Design review of the part built by this model. Coordinates are the model's own, in mm. Give positions to 0.01 mm unless a question says otherwise; leave off trailing zeros. Loops run counter-clockwise (first coordinate to the right, second up) from the corner with the lowest first, then second, coordinate; pieces in that order, holes last. Notation, with made-up numbers: (53.25, 64) - (100.25, 64) arc R19 cw to (100.25, 77) - close; hole circle Ø8 at (73.25, 37). An arc over 180 degrees is marked (long way). Write each question's results on one line, items separated by ' | '.
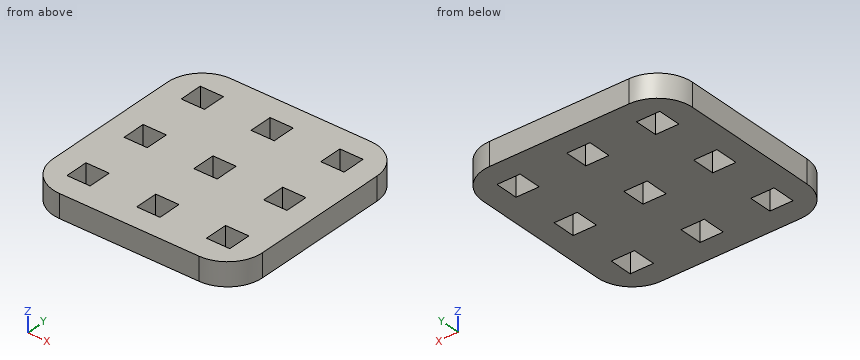
from build123d import *

# Parameters (mm, degrees)
MODEL_W                 = 3
MODEL_H                 = 3
SALIENTE_EXTRUIR1_DEPTH = 3


with BuildPart() as part:
    # Model → Saliente-Extruir1 (new body)
    with BuildSketch(Plane.XY):
        with BuildLine():
            Line((12.895467255, 298.259658236), (30.895467255, 298.259658236))
            ThreePointArc((30.895467255, 298.259658236), (34.077447771, 296.941638751), (35.395467255, 293.759658236))
            Line((35.395467255, 293.759658236), (35.395467255, 275.759658236))
            ThreePointArc((35.395467255, 275.759658236), (34.077447771, 272.577677721), (30.895467255, 271.259658236))
            Line((30.895467255, 271.259658236), (12.895467255, 271.259658236))
            ThreePointArc((12.895467255, 271.259658236), (9.71348674, 272.577677721), (8.395467255, 275.759658236))
            Line((8.395467255, 275.759658236), (8.395467255, 293.759658236))
            ThreePointArc((8.395467255, 293.759658236), (9.71348674, 296.941638751), (12.895467255, 298.259658236))
        make_face()
        with Locations((12.895467255, 293.759658236)):
            Rectangle(MODEL_W, MODEL_H, mode=Mode.SUBTRACT)
        with Locations((21.895467255, 293.759658236)):
            Rectangle(MODEL_W, MODEL_H, mode=Mode.SUBTRACT)
        with Locations((30.895467255, 293.759658236)):
            Rectangle(MODEL_W, MODEL_H, mode=Mode.SUBTRACT)
        with Locations((12.895467255, 275.759658236)):
            Rectangle(MODEL_W, MODEL_H, mode=Mode.SUBTRACT)
        with Locations((21.895467255, 275.759658236)):
            Rectangle(MODEL_W, MODEL_H, mode=Mode.SUBTRACT)
        with Locations((30.895467255, 275.759658236)):
            Rectangle(MODEL_W, MODEL_H, mode=Mode.SUBTRACT)
        with Locations((12.895467255, 284.759658236)):
            Rectangle(MODEL_W, MODEL_H, mode=Mode.SUBTRACT)
        with Locations((21.895467255, 284.759658236)):
            Rectangle(MODEL_W, MODEL_H, mode=Mode.SUBTRACT)
        with Locations((30.895467255, 284.759658236)):
            Rectangle(MODEL_W, MODEL_H, mode=Mode.SUBTRACT)
    extrude(amount=SALIENTE_EXTRUIR1_DEPTH)


solid = part.part
(1) Take a section at B-B on x = 20.75. Give the boundary of the cut face in (y, z), plus the area to 3 significant figures.
Answers below:
outline: (271.26, 0) - (274.26, 0) - (274.26, 3) - (271.26, 3) - close; (277.26, 0) - (283.26, 0) - (283.26, 3) - (277.26, 3) - close; (286.26, 0) - (292.26, 0) - (292.26, 3) - (286.26, 3) - close; (295.26, 0) - (298.26, 0) - (298.26, 3) - (295.26, 3) - close | area: 54.0 mm2
(2) Wall thickness on line 1 along Y through (x, z) = (22, 2.6); line 2 along X through (y, z) = (276.75, 2.25); line 3 along X through (y, z) = (274.5, 0.4): over which ranges is each line inside the solid? List them lowest first. Write a range as from..to.
Answers below:
line 1: 271.26..274.26, 277.26..283.26, 286.26..292.26, 295.26..298.26 | line 2: 8.4..11.4, 14.4..20.4, 23.4..29.4, 32.4..35.4 | line 3: 8.58..11.4, 14.4..20.4, 23.4..29.4, 32.4..35.22
(3) Take a section at C-C on z = 2.4. Count the separate pieces of the cut face and the enclosed holes in it, plus the area to 3 significant figures.
Answers below:
separate pieces: 1 | enclosed holes: 9 | area: 631 mm2
(4) Take a section at A-A on y = 285.5. Give the boundary of the cut face in (x, z).
Answers below:
outline: (8.4, 0) - (11.4, 0) - (11.4, 3) - (8.4, 3) - close; (14.4, 0) - (20.4, 0) - (20.4, 3) - (14.4, 3) - close; (23.4, 0) - (29.4, 0) - (29.4, 3) - (23.4, 3) - close; (32.4, 0) - (35.4, 0) - (35.4, 3) - (32.4, 3) - close
(5) Take a section at D-D on x = 33.5. Give the boundary of the cut face in (y, z), plus the area to 3 significant figures.
Answers below:
outline: (272.09, 0) - (297.43, 0) - (297.43, 3) - (272.09, 3) - close | area: 76.0 mm2
